Verification items for the finished model (mm, model axes). Face numbers are marked on the shaded views. Coordinates: 2 decimals unless noted, no trailing zeros. Order: outer loops, then holes, each group sorted by start corner. A loop starts at its lowest first (then second) coordinate and runs counter-clockwise, first axis right, second up.
Q1. Thickness scan on line 1 (Y direction, x = -19, z = 4.45); line 2 (X direction, y = -14.5, z = 2). Record the ranges inside material, lowest first.
Q2. Cross-section at D-D, the plane z = 1.05. Record the boundary of the cut face in (x, y), and give its area (3 significant figures).
Q3. Depth check by flat-ended pin: P1, Ø12, axis at x = -5.5, y = -13, coming from the -Z side; P2, Ø8, axis at x = 19, y = -19, coming from the +Z side. Enter the tip coordinate at first touch or a pass-through.
Q4. Draft check along Y on the marked faces 1, 2 and 3. Enter one of: pulls with the +Y half, pulls with the -Y half, needs draft (parallel to the pull), parting line crosses it, or undercut.
Q5. Cross-section at A-A, the plane y = 19. Record the boundary of the cut face in (x, z), and give its area (3 significant figures).
Q6. Cross-section at C-C, the plane x = 0. Record the boundary of the cut face in (y, z).
Autodesk Inventor part; units mm, degrees
ref_plane "YZ Plane" through (0, 0, 0) normal (1, 0, 0) x (0, 1, 0)
ref_plane "XZ Plane" through (0, 0, 0) normal (0, 1, 0) x (-1, 0, 0)
ref_plane "XY Plane" through (0, 0, 0) normal (0, 0, 1) x (1, 0, 0)
sketch "Schizzo1" plane through (0, 0, 0) normal (0, 0, 1) x (1, 0, 0)
  line L0 (-30, 30) -> (30, 30)
  line L1 (30, 30) -> (30, -30)
  line L2 (30, -30) -> (-30, -30)
  line L3 (-30, -30) -> (-30, 30)
  line L4 (-30, 30) -> (30, -30) construction
  line L5 (30, 30) -> (-30, -30) construction
  circle A0 centre (0, 0) radius 5
  dimension "d0" = 60
  dimension "d1" = 60
  dimension "d5" = 10
extrude "Estrusione2" add sketch "Schizzo1" along normal blind 5
fillet "Raccordo2" radius 5 4 edges at (-30, 30, 2.5) (30, 30, 2.5) (30, -30, 2.5) (-30, -30, 2.5)
sketch "Schizzo3" plane through (0, 0, 5) normal (0, 0, 1) x (1, 0, 0)
  circle A0 centre (19, -19) radius 6.4
  circle A1 centre (-19, -19) radius 4.5
  circle A2 centre (19, 19) radius 4.5
  circle A3 centre (-19, 19) radius 3
  point P0 (0, 0)
hole "Foro1" at (19, -19, 5) at (19, 19, 5) at (-19, 19, 5) at (-19, -19, 5) direction (0, 0, -1) diameter 10 end through all
properties part number "Piastra supporto pistone lama"
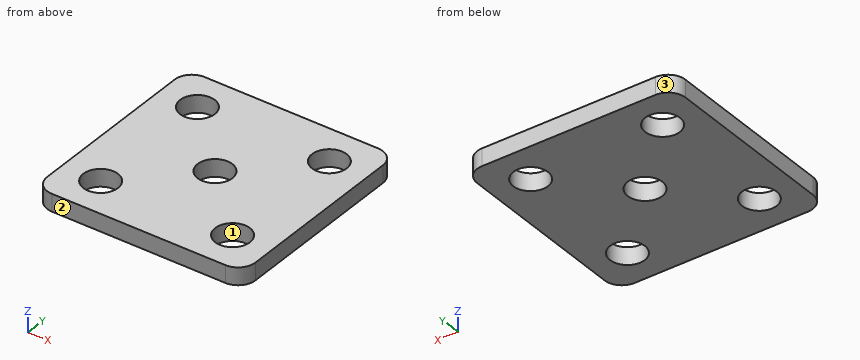
Check values:
1. line 1: y = -30 to -24, -14 to 14, 24 to 30
1. line 2: x = -30 to -21.18, -16.82 to 16.82, 21.18 to 30
2. outline: (-30, -25) arc R5 ccw to (-25, -30) - (25, -30) arc R5 ccw to (30, -25) - (30, 25) arc R5 ccw to (25, 30) - (-25, 30) arc R5 ccw to (-30, 25) - close; hole circle Ø10 at (-19, -19); hole circle Ø10 at (-19, 19); hole circle Ø10 at (0, 0); hole circle Ø10 at (19, -19); hole circle Ø10 at (19, 19)
2. area: 3,190 mm2
3. P1: stops at z = 0
3. P2: passes through
4. face 1: undercut
4. face 2: pulls with the -Y half
4. face 3: pulls with the +Y half
5. outline: (-30, 0) - (-24, 0) - (-24, 5) - (-30, 5) - close; (-14, 0) - (14, 0) - (14, 5) - (-14, 5) - close; (24, 0) - (30, 0) - (30, 5) - (24, 5) - close
5. area: 200 mm2
6. outline: (-30, 0) - (-5, 0) - (-5, 5) - (-30, 5) - close; (5, 0) - (30, 0) - (30, 5) - (5, 5) - close
